Work out the finished part from the listing and answer in its coordinate system (mm). Face numbers are marked on the shaded views. A direction names the side the tool comes from. Coordinates: 2 decimals unless noted, no trailing zeros. Loops run counter-clockwise (first coordinate to the right, second up) from the corner with the lowest first, then second, coordinate; pieces in that order, holes last. Notation, with made-up numbers: (53.25, -10) -> (96.25, -10) arc R19 cw to (96.25, 24) -> close; hole circle Ø11 at (76, 10.5). An arc over 180 degrees is marked (long way). One line per question, with ' | ' between items.
```python
from build123d import *

# Parameters (mm, degrees)
SKETCH_W          = 25
SKETCH_H          = 40
PAD_DEPTH         = 20
SKETCH001_R       = 3.8
PAD001_DEPTH      = 17
PAD001_DEPTH_BACK = 34
SKETCH002_R       = 5
PAD002_DEPTH      = 10
PAD002_DEPTH_BACK = 27
SKETCH003_W       = 14.2
SKETCH003_H       = 14.2
POCKET_DEPTH      = 50
FILLET003_R       = 3
FILLET004_R       = 1


with BuildPart() as part:
    # Sketch → Pad (new body)
    with BuildSketch(Plane.XY):
        Rectangle(SKETCH_W, SKETCH_H)
    extrude(amount=PAD_DEPTH)

    # Sketch001 → Pad001 (new body, two sides)
    with BuildSketch(Plane(origin=(-12.5, 0, 0), x_dir=(0, -1, 0), z_dir=(-1, 0, 0))) as pad001_sk:
        with Locations((0, 10)):
            Circle(SKETCH001_R)
    extrude(amount=PAD001_DEPTH)
    extrude(pad001_sk.sketch, amount=-PAD001_DEPTH_BACK)

    # Sketch002 → Pad002 (new body, two sides)
    with BuildSketch(Plane(origin=(-12.5, 0, 0), x_dir=(0, -1, 0), z_dir=(-1, 0, 0))) as pad002_sk:
        with Locations((0, 10)):
            Circle(SKETCH002_R)
    extrude(amount=PAD002_DEPTH)
    extrude(pad002_sk.sketch, amount=-PAD002_DEPTH_BACK)

    # Sketch003 → Pocket (cut)
    with BuildSketch(Plane.XZ.offset(20)):
        with Locations((0, 7.1)):
            Rectangle(SKETCH003_W, SKETCH003_H)
    extrude(amount=-POCKET_DEPTH, mode=Mode.SUBTRACT)

    # Fillet003
    fillet003_edges = [part.edges().sort_by_distance(p)[0] for p in [
        (-12.5, 5, 10),
    ]]
    fillet(fillet003_edges, radius=FILLET003_R)

    # Fillet004
    fillet004_edges = [part.edges().sort_by_distance(p)[0] for p in [
        (12.5, 5, 10),
    ]]
    fillet(fillet004_edges, radius=FILLET004_R)


solid = part.part
```
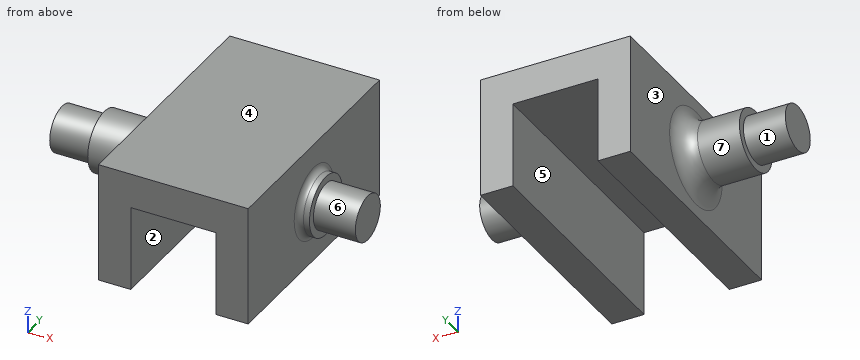
1) Find section C-C (x = -24). Write down the section's boundary in (y, z).
Check values:
outline: circle Ø7.6 at (0, 10)
2) Find section A-A (z = 10). Write down the section's boundary in (x, y), plus the area to 3 significant figures.
Check values:
outline: (-29.5, -3.8) -> (-22.5, -3.8) -> (-22.5, -5) -> (-15.5, -5) arc R3 cw to (-12.5, -8) -> (-12.5, -20) -> (-7.1, -20) -> (-7.1, 20) -> (-12.5, 20) -> (-12.5, 8) arc R3 cw to (-15.5, 5) -> (-22.5, 5) -> (-22.5, 3.8) -> (-29.5, 3.8) -> close; (7.1, -20) -> (12.5, -20) -> (12.5, -6) arc R1 cw to (13.5, -5) -> (14.5, -5) -> (14.5, -3.8) -> (21.5, -3.8) -> (21.5, 3.8) -> (14.5, 3.8) -> (14.5, 5) -> (13.5, 5) arc R1 cw to (12.5, 6) -> (12.5, 20) -> (7.1, 20) -> close | area: 663 mm^2
3) Find section B-B (y = 9). Write down the section's boundary in (x, z).
Check values:
outline: (-12.5, 0) -> (-7.1, 0) -> (-7.1, 14.2) -> (7.1, 14.2) -> (7.1, 0) -> (12.5, 0) -> (12.5, 20) -> (-12.5, 20) -> close
4) For the marked faces 4, 5, 6 and 7, determine the directions among +Z, -Z, +X, -X, +Y, -Y from which every point of the face is accessible in a straight line to the end or side of a thin tool.
Check values:
face 4: +Z, +X, -X, +Y, -Y | face 5: -Z, +Y, -Y | face 6: +X | face 7: -X
5) The mould has two halves that part along X. Classify the marked faces 1, 2 and 3: released by +X, released by -X, zero draft, split by the parting line, or undercut.
Check values:
face 1: zero draft | face 2: undercut | face 3: released by -X
6) Find the intervals of material crossed by line 1 along X through (y, z) = (-9, 5.5); line 2 along X through (y, z) = (8.5, 16); line 3 along Z through (x, y) = (7, 14), in increasing order.
Check values:
line 1: x = -12.5 to -7.1, 7.1 to 12.5 | line 2: x = -12.5 to 12.5 | line 3: z = 14.2 to 20
7) Flat-ended cylindrical pins translate along their axes: pin 1 (10 mm diameter, centred on x = -20.5, z = 13.5, fed in from +Y); pin 2 (4 mm diameter, centred on y = -14, z = 9, fed in from +X); pin 3 (1.5 mm diameter, centred on y = -3.5, z = 13.5, fed in from +X). Find the tip coordinate at first contact, or state that the pin passes through.
Check values:
pin 1: stops at y = 5 | pin 2: stops at x = 12.5 | pin 3: stops at x = 14.5
8) Find section D-D (y = 0). Write down the section's boundary in (x, z).
Check values:
outline: (-29.5, 6.2) -> (-22.5, 6.2) -> (-22.5, 5) -> (-15.5, 5) arc R3 cw to (-12.5, 2) -> (-12.5, 0) -> (-7.1, 0) -> (-7.1, 14.2) -> (7.1, 14.2) -> (7.1, 0) -> (12.5, 0) -> (12.5, 4) arc R1 cw to (13.5, 5) -> (14.5, 5) -> (14.5, 6.2) -> (21.5, 6.2) -> (21.5, 13.8) -> (14.5, 13.8) -> (14.5, 15) -> (13.5, 15) arc R1 cw to (12.5, 16) -> (12.5, 20) -> (-12.5, 20) -> (-12.5, 18) arc R3 cw to (-15.5, 15) -> (-22.5, 15) -> (-22.5, 13.8) -> (-29.5, 13.8) -> close
